Part model, mm, in its own coordinate system. A direction names the side the tool comes from. Give positions to 0.01 mm unless a question says otherwise; leave off trailing zeros. Write each loop counter-clockwise with the first axis right and the second up, starting at its lowest first coordinate (ties: lowest second). Pieces come first, ordered by that corner, then holes. Notation, with made-up numbers: (-8.5, -31.75) - (-4.5, -31.75) arc R32 cw to (-4.5, -0.75) - close; hole circle Ø4 at (44, 66). An arc over 180 degrees is marked (long way). Answer as a JSON object with one key per item and string values. Group by question number.
Autodesk Inventor part; units mm, degrees
ref_plane "YZ Plane" through (0, 0, 0) normal (1, 0, 0) x (0, 1, 0)
ref_plane "XZ Plane" through (0, 0, 0) normal (0, 1, 0) x (-1, 0, 0)
ref_plane "XY Plane" through (0, 0, 0) normal (0, 0, 1) x (1, 0, 0)
sketch "Boceto1" plane through (0, 0, 0) normal (0, 0, 1) x (1, 0, 0)
  arc A0 (-18.1173, 21.3488) -> (-19.6673, 19.7988) centre (-18.1173, 19.7988) ccw
  arc A1 (-19.6673, 19.7988) -> (-18.1173, 18.2488) centre (-18.1173, 19.7988) ccw
  arc A2 (-18.1173, 18.2488) -> (-16.5673, 19.7988) centre (-18.1173, 19.7988) ccw
  arc A3 (-16.5673, 19.7988) -> (-18.1173, 21.3488) centre (-18.1173, 19.7988) ccw
  arc A4 (-18.1173, -7.6512) -> (-19.6673, -9.2012) centre (-18.1173, -9.2012) ccw
  arc A5 (-19.6673, -9.2012) -> (-18.1173, -10.7512) centre (-18.1173, -9.2012) ccw
  arc A6 (-18.1173, -10.7512) -> (-16.5673, -9.2012) centre (-18.1173, -9.2012) ccw
  arc A7 (-16.5673, -9.2012) -> (-18.1173, -7.6512) centre (-18.1173, -9.2012) ccw
  arc A8 (-18.1173, -36.6512) -> (-19.6673, -38.2012) centre (-18.1173, -38.2012) ccw
  arc A9 (-19.6673, -38.2012) -> (-18.1173, -39.7512) centre (-18.1173, -38.2012) ccw
  arc A10 (-18.1173, -39.7512) -> (-16.5673, -38.2012) centre (-18.1173, -38.2012) ccw
  arc A11 (-16.5673, -38.2012) -> (-18.1173, -36.6512) centre (-18.1173, -38.2012) ccw
  arc A12 (-67.1173, 21.3488) -> (-68.6673, 19.7988) centre (-67.1173, 19.7988) ccw
  arc A13 (-68.6673, 19.7988) -> (-67.1173, 18.2488) centre (-67.1173, 19.7988) ccw
  arc A14 (-67.1173, 18.2488) -> (-65.5673, 19.7988) centre (-67.1173, 19.7988) ccw
  arc A15 (-65.5673, 19.7988) -> (-67.1173, 21.3488) centre (-67.1173, 19.7988) ccw
  arc A16 (-67.1173, -3.6326) -> (-68.6673, -5.1826) centre (-67.1173, -5.1826) ccw
  arc A17 (-68.6673, -5.1826) -> (-67.1173, -6.7326) centre (-67.1173, -5.1826) ccw
  arc A18 (-67.1173, -6.7326) -> (-65.5673, -5.1826) centre (-67.1173, -5.1826) ccw
  arc A19 (-65.5673, -5.1826) -> (-67.1173, -3.6326) centre (-67.1173, -5.1826) ccw
  arc A20 (-72.6173, -36.6512) -> (-74.1673, -38.2012) centre (-72.6173, -38.2012) ccw
  arc A21 (-74.1673, -38.2012) -> (-72.6173, -39.7512) centre (-72.6173, -38.2012) ccw
  arc A22 (-72.6173, -39.7512) -> (-71.0673, -38.2012) centre (-72.6173, -38.2012) ccw
  arc A23 (-71.0673, -38.2012) -> (-72.6173, -36.6512) centre (-72.6173, -38.2012) ccw
  arc A24 (-116.1173, 21.3488) -> (-117.6673, 19.7988) centre (-116.1173, 19.7988) ccw
  arc A25 (-117.6673, 19.7988) -> (-116.1173, 18.2488) centre (-116.1173, 19.7988) ccw
  arc A26 (-116.1173, 18.2488) -> (-114.5673, 19.7988) centre (-116.1173, 19.7988) ccw
  arc A27 (-114.5673, 19.7988) -> (-116.1173, 21.3488) centre (-116.1173, 19.7988) ccw
  arc A28 (-116.1173, -7.6512) -> (-117.6673, -9.2012) centre (-116.1173, -9.2012) ccw
  arc A29 (-117.6673, -9.2012) -> (-116.1173, -10.7512) centre (-116.1173, -9.2012) ccw
  arc A30 (-116.1173, -10.7512) -> (-114.5673, -9.2012) centre (-116.1173, -9.2012) ccw
  arc A31 (-114.5673, -9.2012) -> (-116.1173, -7.6512) centre (-116.1173, -9.2012) ccw
  arc A32 (-116.1173, -36.6512) -> (-117.6673, -38.2012) centre (-116.1173, -38.2012) ccw
  arc A33 (-117.6673, -38.2012) -> (-116.1173, -39.7512) centre (-116.1173, -38.2012) ccw
  arc A34 (-116.1173, -39.7512) -> (-114.5673, -38.2012) centre (-116.1173, -38.2012) ccw
  arc A35 (-114.5673, -38.2012) -> (-116.1173, -36.6512) centre (-116.1173, -38.2012) ccw
  arc A36 (-107.1173, -22.7512) -> (-112.0673, -27.7012) centre (-107.1173, -27.7012) ccw
  arc A37 (-112.0673, -27.7012) -> (-107.1173, -32.6512) centre (-107.1173, -27.7012) ccw
  arc A38 (-107.1173, -32.6512) -> (-102.1673, -27.7012) centre (-107.1173, -27.7012) ccw
  arc A39 (-102.1673, -27.7012) -> (-107.1173, -22.7512) centre (-107.1173, -27.7012) ccw
  arc A40 (-27.1173, -22.7512) -> (-32.0673, -27.7012) centre (-27.1173, -27.7012) ccw
  arc A41 (-32.0673, -27.7012) -> (-27.1173, -32.6512) centre (-27.1173, -27.7012) ccw
  arc A42 (-27.1173, -32.6512) -> (-22.1673, -27.7012) centre (-27.1173, -27.7012) ccw
  arc A43 (-22.1673, -27.7012) -> (-27.1173, -22.7512) centre (-27.1173, -27.7012) ccw
  line L0 (-83.2173, 1.8988) -> (-83.2173, 12.6988)
  line L1 (-83.2173, 12.6988) -> (-112.0173, 12.6988)
  line L2 (-112.0173, 12.6988) -> (-112.0173, 1.8988)
  line L3 (-112.0173, 1.8988) -> (-83.2173, 1.8988)
  line L4 (-22.2173, 1.8988) -> (-22.2173, 12.6988)
  line L5 (-22.2173, 12.6988) -> (-51.0173, 12.6988)
  line L6 (-51.0173, 12.6988) -> (-51.0173, 1.8988)
  line L7 (-51.0173, 1.8988) -> (-22.2173, 1.8988)
  line L8 (-67.4673, -14.8512) -> (-37.6673, -14.8512)
  line L9 (-37.6673, -14.8512) -> (-37.6673, -42.8512)
  line L10 (-37.6673, -42.8512) -> (-11.9673, -42.8512)
  line L11 (-11.9673, -42.8512) -> (-11.9673, 27.4488)
  line L12 (-11.9673, 27.4488) -> (-122.2673, 27.4488)
  line L13 (-122.2673, 27.4488) -> (-122.2673, -42.8512)
  line L14 (-122.2673, -42.8512) -> (-67.4673, -42.8512)
  line L15 (-67.4673, -42.8512) -> (-67.4673, -14.8512)
  point P0 (0, 0)
extrude "Extrusión1" add sketch "Boceto1" along normal blind 5
properties part number "carro x lado polea pieza4 tapa"
1) Band-saw the part on C-C (z = 2.15). State how many separate pieces and enclosed holes the cut face has, plus the area to 3 significant figures.
2) Band-saw the part on B-B (x = -43). List the corners of the cut face in (y, z), plus the area to 4 significant figures.
3) Band-saw the part on A-A (y = 11.5). List the corners of the cut face in (x, z), plus the area to 4 significant figures.
4) Probe line 1 (X direction, y = 4, z = 3.4); line 2 (Y direction, x = -110.5, z = 3.5); line 3 (Y direction, x = -35, z = 2.95). List the from-to ranges inside material, lowest first.
5) Band-saw the part on D-D (x = -104.5). List the corners of the cut face in (y, z), plus the area to 3 significant figures.
6) Which spindle directions (+Z, -Z, +X, -X, +Y, -Y) get a long thin tool onto all of the face, cutting with end or side? Do faces 5 (the flat face through (-51.017, 7, 2)), 6 (the flat face through (-37.667, -29, 2)), 7 (the flat face through (-68, -7, 5)). Say none if no direction does.
7) Mould opens along X. For faces 1 (the cylindrical face through (-65.64, -5.65, 2.46)), 2 (the cylindrical face through (-114.57, 19.87, 2.46)), 3 (the flat face through (-66, 27.449, 2)), 4 (the flat face through (-11.967, -8, 2)) say: pulls with the +X half, pulls with the -X half, needs draft (parallel to the pull), parting line crosses it, or undercut.
Verdict:
{
 "1": {"separate pieces": "1", "enclosed holes": "13", "area": "6,080 mm2"},
 "2": {"outline": "(-14.85, 0) - (1.9, 0) - (1.9, 5) - (-14.85, 5) - close; (12.7, 0) - (27.45, 0) - (27.45, 5) - (12.7, 5) - close", "area": "157.5 mm2"},
 "3": {"outline": "(-122.27, 0) - (-112.02, 0) - (-112.02, 5) - (-122.27, 5) - close; (-83.22, 0) - (-51.02, 0) - (-51.02, 5) - (-83.22, 5) - close; (-22.22, 0) - (-11.97, 0) - (-11.97, 5) - (-22.22, 5) - close", "area": "263.5 mm2"},
 "4": {"line 1": "-122.27 to -112.02, -83.22 to -51.02, -22.22 to -11.97", "line 2": "-42.85 to -31.32, -24.09 to 1.9, 12.7 to 27.45", "line 3": "-42.85 to 1.9, 12.7 to 27.45"},
 "5": {"outline": "(-42.85, 0) - (-31.9, 0) - (-31.9, 5) - (-42.85, 5) - close; (-23.5, 0) - (1.9, 0) - (1.9, 5) - (-23.5, 5) - close; (12.7, 0) - (27.45, 0) - (27.45, 5) - (12.7, 5) - close", "area": "255 mm2"},
 "6": {"face 5": "+Z, -Z", "face 6": "+Z, -Z, -Y", "face 7": "+Z, +X, -X, +Y, -Y"},
 "7": {"face 1": "undercut", "face 2": "undercut", "face 3": "needs draft", "face 4": "pulls with the +X half"}
}
